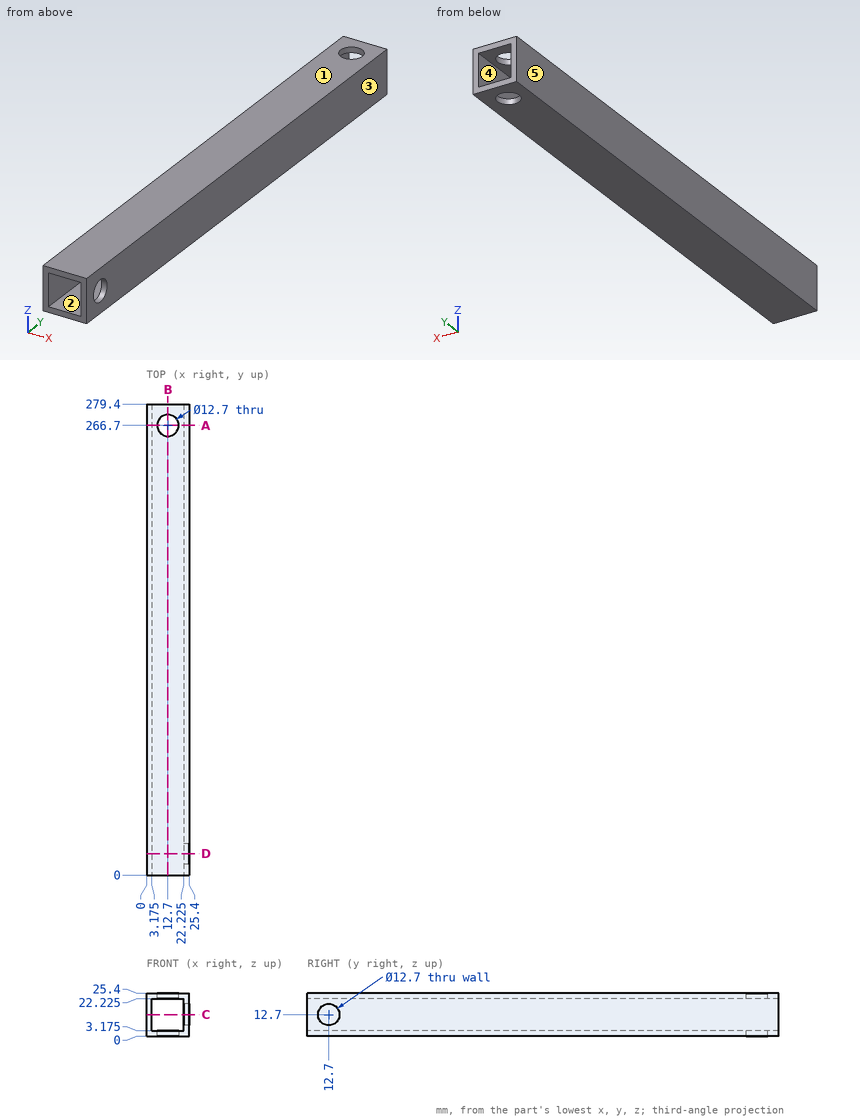
Source: three-view drawing plus pictorial views. Frame: mm from the lowest corner of the part. A direction names the side the tool comes from. Round coordinates to 2 decimals unless told otherwise and drop trailing zeros. Loops run counter-clockwise (first coordinate to the right, second up) from the corner with the lowest first, then second, coordinate; pieces in that order, holes last.
Q1. Section D-D on y = 12.7. Return loops of the section in (x, z) (3 decimals).
Q2. Section C-C on z = 12.7. Return loops of the section in (x, y) (3 decimals), plus the area to 3 significant figures.
Q3. Section B-B on x = 12.7. Return loops of the section in (y, z) (3 decimals).
Q4. Material intervals for L1, parallel to Z at x = 14.25, y = 67 (3 decimals); L2, parallel to X at y = 266.7, z = 2.15, sorted ascending.
Q5. Pin query (flat end, axial travel): P1, Ø12, axis at x = 14, z = 13, coming from the -Y side. Return the tip coordinate at first contact, or that it passes through.
Q6. Section A-A on y = 266.7. Return loops of the section in (x, z) (3 decimals).
Q7. Pull-direction query (X, two-part tool) for the marked faces 1, 2 and 3; classes: released by +X, released by -X, zero draft, split by the parting line, or undercut.
Q8. Access query for the marked faces 4 and 5. Directions: +Z, -Z, +X, -X, +Y, -Y. A direction counts if a zero-diameter tool reaches every point of the face in a straight line with its end or side. Return the directions, or none.
Evaluation:
1. outline: (0, 0) - (25.4, 0) - (25.4, 6.35) - (22.225, 6.35) - (22.225, 3.175) - (3.175, 3.175) - (3.175, 22.225) - (22.225, 22.225) - (22.225, 19.05) - (25.4, 19.05) - (25.4, 25.4) - (0, 25.4) - close
2. outline: (0, 0) - (3.175, 0) - (3.175, 279.4) - (0, 279.4) - close; (22.225, 0) - (25.4, 0) - (25.4, 6.35) - (22.225, 6.35) - close; (22.225, 19.05) - (25.4, 19.05) - (25.4, 279.4) - (22.225, 279.4) - close
2. area: 1,730 mm2
3. outline: (0, 0) - (260.35, 0) - (260.35, 3.175) - (0, 3.175) - close; (0, 22.225) - (260.35, 22.225) - (260.35, 25.4) - (0, 25.4) - close; (273.05, 0) - (279.4, 0) - (279.4, 3.175) - (273.05, 3.175) - close; (273.05, 22.225) - (279.4, 22.225) - (279.4, 25.4) - (273.05, 25.4) - close
4. L1: z = 0 to 3.175, 22.225 to 25.4
4. L2: x = 0 to 6.35, 19.05 to 25.4
5. P1: passes through
6. outline: (0, 0) - (6.35, 0) - (6.35, 3.175) - (3.175, 3.175) - (3.175, 22.225) - (6.35, 22.225) - (6.35, 25.4) - (0, 25.4) - close; (19.05, 0) - (25.4, 0) - (25.4, 25.4) - (19.05, 25.4) - (19.05, 22.225) - (22.225, 22.225) - (22.225, 3.175) - (19.05, 3.175) - close
7. face 1: zero draft
7. face 2: undercut
7. face 3: released by +X
8. face 4: +Y, -Y
8. face 5: +Z, -Z, -X, +Y, -Y
